Study the drawing (mm; zero at the part's minimum x, y, z) and answer. Round coordinates to 2 decimals unless told otherwise and drop trailing zeros. Loops run counter-clockwise (first coordinate to the right, second up) from the corner with the lowest first, then second, coordinate; pieces in that order, holes last. Notation, with made-up numbers: M -1.75,25.5 L 41.25,25.5 A20 ccw 41.25,46.5 Z; hole C 72,67 d5. An arc over 180 degrees is marked long. Write each question's results on one line, items separated by ' | '.
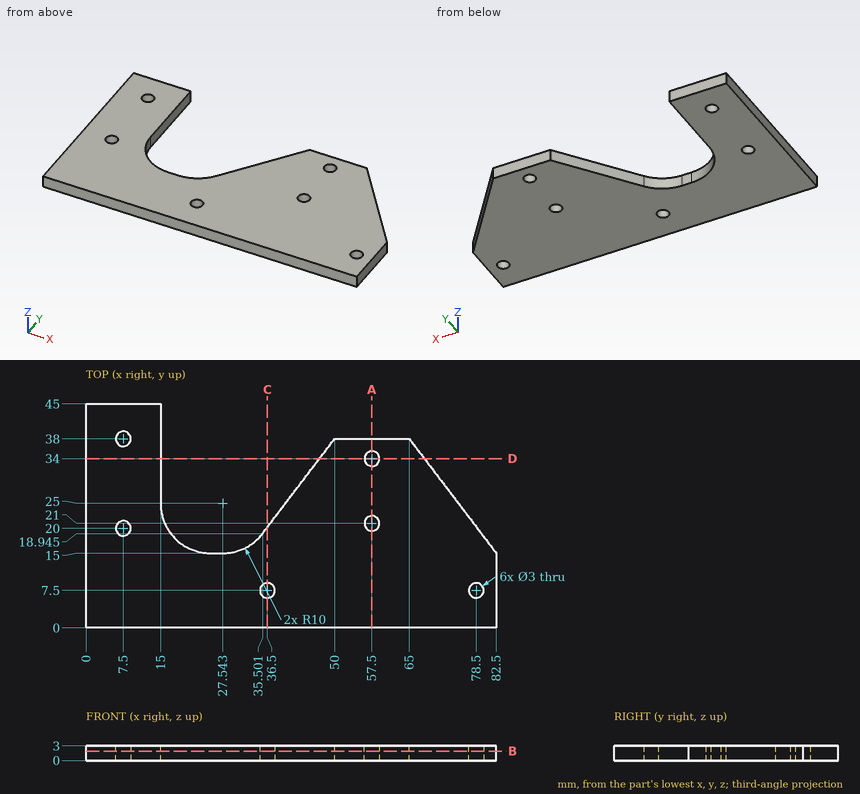
Item 1: The part is cut by section D-D (y = 34). Determine the outline of the cut face in (x, z).
Outcome:
outline: M 0,0 L 15,0 L 15,3 L 0,3 Z; M 46.96,0 L 56,0 L 56,3 L 46.96,3 Z; M 59,0 L 68.04,0 L 68.04,3 L 59,3 Z
Item 2: The part is cut by section C-C (x = 36.5). Determine the outline of the cut face in (y, z).
Outcome:
outline: M 0,0 L 6,0 L 6,3 L 0,3 Z; M 9,0 L 20.26,0 L 20.26,3 L 9,3 Z
Item 3: The part is cut by section A-A (x = 57.5). Determine the outline of the cut face in (y, z).
Outcome:
outline: M 0,0 L 19.5,0 L 19.5,3 L 0,3 Z; M 22.5,0 L 32.5,0 L 32.5,3 L 22.5,3 Z; M 35.5,0 L 38,0 L 38,3 L 35.5,3 Z
Item 4: Flat-ended cylindrical pins translate along their axes: pin 1 (1.5 mm diameter, centred on x = 43, z = 2.5, fed in from +Y) (1 decimal); pin 2 (1.8 mm diameter, centred on x = 7.5, y = 20, fed in from +Z); pin 3 (1.5 mm diameter, centred on x = 54.5, z = 1.5, fed in from +Y). Find the tip coordinate at first contact, or state that the pin passes through.
Outcome:
pin 1: stops at y = 29.8 | pin 2: passes through | pin 3: stops at y = 38
Item 5: Straight lines are drawn through the part: line 1 (X direction, y = 20.5, z = 1.95) (1 decimal); line 2 (X direction, y = 37, z = 2); line 3 (Y direction, x = 7.5, z = 0.2). For each, find the intervals that lie inside material, in ascending order.
Outcome:
line 1: x = 0 to 6.1, 8.9 to 16.1, 36.7 to 56.1, 58.9 to 78.3 | line 2: x = 0 to 6.38, 8.62 to 15, 49.24 to 65.76 | line 3: y = 0 to 18.5, 21.5 to 36.5, 39.5 to 45
Item 6: The part is cut by section B-B (z = 1.9). Determine the outline of the cut face in (x, y) (1 decimal), plus the area to 3 significant figures.
Outcome:
outline: M 0,0 L 82.5,0 L 82.5,15 L 65,38 L 50,38 L 35.5,18.9 A10 cw 27.5,15 L 25,15 A10 cw 15,25 L 15,45 L 0,45 Z; hole C 7.5,20 d3; hole C 7.5,38 d3; hole C 36.5,7.5 d3; hole C 57.5,21 d3; hole C 57.5,34 d3; hole C 78.5,7.5 d3 | area: 2,420 mm2
